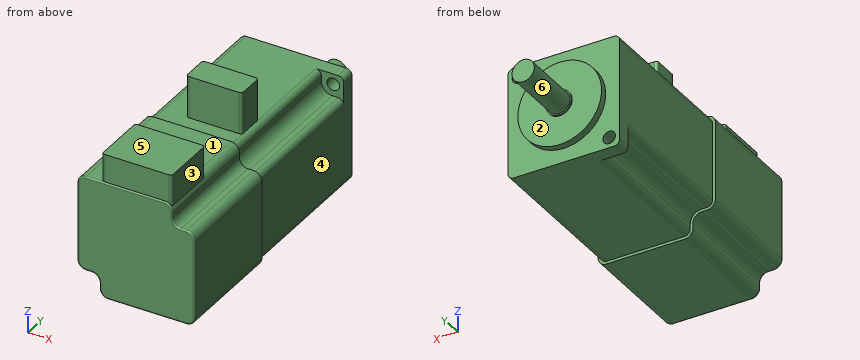
```python
from build123d import *

# Parameters (mm, degrees)
BOSS_EXTRUDE1_DEPTH             = 5
SKETCH2_R                       = 15
BOSS_EXTRUDE2_DEPTH             = 2.5
SKETCH3_R                       = 2.25
CUT_EXTRUDE1_DEPTH              = 5
BOSS_EXTRUDE3_DEPTH             = 51
BOSS_EXTRUDE4_DEPTH             = 40.5
SKETCH6_R                       = 4.5
BOSS_EXTRUDE5_DEPTH             = 0.5
SKETCH7_R                       = 4
BOSS_EXTRUDE6_DEPTH             = 21.5
FILLET1_R                       = 0.5
BOSS_EXTRUDE7_DEPTH             = 15
BOSS_EXTRUDE8_DEPTH             = 10
BOSS_EXTRUDE8_DIRECTION_2_REACH = 44


with BuildPart() as part:
    # Sketch1 → Boss-Extrude1 (new body)
    with BuildSketch(Plane(origin=(0, 0, 0), x_dir=(1, 0, 0), z_dir=(0, 1, 0))):
        with BuildLine():
            Line((2, 0), (38, 0))
            ThreePointArc((38, 0), (39.414213562, 0.585786438), (40, 2))
            Line((40, 2), (40, 38))
            ThreePointArc((40, 38), (39.414213562, 39.414213562), (38, 40))
            Line((38, 40), (2, 40))
            ThreePointArc((2, 40), (0.585786438, 39.414213562), (0, 38))
            Line((0, 38), (0, 2))
            ThreePointArc((0, 2), (0.585786438, 0.585786438), (2, 0))
        make_face()
    extrude(amount=BOSS_EXTRUDE1_DEPTH)

    # Sketch2 → Boss-Extrude2 (add)
    with BuildSketch(Plane(origin=(0, 5, 0), x_dir=(1, 0, 0), z_dir=(0, 1, 0))):
        with Locations((20, 20)):
            Circle(SKETCH2_R)
    extrude(amount=BOSS_EXTRUDE2_DEPTH)

    # Sketch3 → Cut-Extrude1 (cut)
    with BuildSketch(Plane(origin=(0, 5, 0), x_dir=(1, 0, 0), z_dir=(0, 1, 0))):
        with Locations((3.736544033, 36.263455967)):
            Circle(SKETCH3_R)
        with Locations((36.263455967, 3.736544033)):
            Circle(SKETCH3_R)
    extrude(amount=-CUT_EXTRUDE1_DEPTH, mode=Mode.SUBTRACT)

    # Sketch4 → Boss-Extrude3 (add)
    with BuildSketch(Plane.XZ):
        with BuildLine():
            Line((32, -2), (32, -4))
            ThreePointArc((32, -4), (33.171572875, -6.828427125), (36, -8))
            Line((36, -8), (38, -8))
            ThreePointArc((38, -8), (39.414213562, -8.585786438), (40, -10))
            Line((40, -10), (40, -38))
            ThreePointArc((40, -38), (39.414213562, -39.414213562), (38, -40))
            Line((38, -40), (10, -40))
            ThreePointArc((10, -40), (8.585786438, -39.414213562), (8, -38))
            Line((8, -38), (8, -36))
            ThreePointArc((8, -36), (6.828427125, -33.171572875), (4, -32))
            Line((4, -32), (2, -32))
            ThreePointArc((2, -32), (0.585786438, -31.414213562), (0, -30))
            Line((0, -30), (0, -2))
            ThreePointArc((0, -2), (0.585786438, -0.585786438), (2, 0))
            Line((2, 0), (30, 0))
            ThreePointArc((30, 0), (31.414213562, -0.585786438), (32, -2))
        make_face()
    extrude(amount=BOSS_EXTRUDE3_DEPTH)

    # Sketch5 → Boss-Extrude4 (add)
    with BuildSketch(Plane.XZ.offset(51)):
        with BuildLine():
            Line((10, -41), (38, -41))
            ThreePointArc((38, -41), (40.121320344, -40.121320344), (41, -38))
            Line((41, -38), (41, -10))
            ThreePointArc((41, -10), (40.121320344, -7.878679656), (38, -7))
            Line((38, -7), (36, -7))
            ThreePointArc((36, -7), (33.878679656, -6.121320344), (33, -4))
            Line((33, -4), (33, -2))
            ThreePointArc((33, -2), (32.121320344, 0.121320344), (30, 1))
            Line((30, 1), (2, 1))
            ThreePointArc((2, 1), (-0.121320344, 0.121320344), (-1, -2))
            Line((-1, -2), (-1, -30))
            ThreePointArc((-1, -30), (-0.121320344, -32.121320344), (2, -33))
            Line((2, -33), (4, -33))
            ThreePointArc((4, -33), (6.121320344, -33.878679656), (7, -36))
            Line((7, -36), (7, -38))
            ThreePointArc((7, -38), (7.878679656, -40.121320344), (10, -41))
        make_face()
    extrude(amount=BOSS_EXTRUDE4_DEPTH)

    # Sketch6 → Boss-Extrude5 (add)
    with BuildSketch(Plane(origin=(0, 7.5, 0), x_dir=(1, 0, 0), z_dir=(0, 1, 0))):
        with Locations((20, 20)):
            Circle(SKETCH6_R)
    extrude(amount=BOSS_EXTRUDE5_DEPTH)

    # Sketch7 → Boss-Extrude6 (add)
    with BuildSketch(Plane(origin=(0, 8, 0), x_dir=(1, 0, 0), z_dir=(0, 1, 0))):
        with Locations((20, 20)):
            Circle(SKETCH7_R)
    extrude(amount=BOSS_EXTRUDE6_DEPTH)

    # Fillet1
    fillet1_edges = [part.edges().sort_by_distance(p)[0] for p in [
        (7.878679656, -91.5, -40.121320344),
        (24, -91.5, -41),
        (40.121320344, -91.5, -40.121320344),
        (41, -91.5, -24),
        (40.121320344, -91.5, -7.878679656),
        (37, -91.5, -7),
        (33.878679656, -91.5, -6.121320344),
        (33, -91.5, -3),
        (32.121320344, -91.5, 0.121320344),
        (16, -91.5, 1),
        (-0.121320344, -91.5, 0.121320344),
        (-1, -91.5, -16),
        (-0.121320344, -91.5, -32.121320344),
        (3, -91.5, -33),
        (6.121320344, -91.5, -33.878679656),
        (7, -91.5, -37),
    ]]
    fillet(fillet1_edges, radius=FILLET1_R)

    # Sketch8 → Boss-Extrude7 (add)
    with BuildSketch(Plane.XY):
        with BuildLine():
            Line((11, -34.5), (29, -34.5))
            ThreePointArc((29, -34.5), (29.707106781, -34.792893219), (30, -35.5))
            Line((30, -35.5), (30, -43.5))
            ThreePointArc((30, -43.5), (29.707106781, -44.207106781), (29, -44.5))
            Line((29, -44.5), (11, -44.5))
            ThreePointArc((11, -44.5), (10.292893219, -44.207106781), (10, -43.5))
            Line((10, -43.5), (10, -35.5))
            ThreePointArc((10, -35.5), (10.292893219, -34.792893219), (11, -34.5))
        make_face()
    extrude(amount=BOSS_EXTRUDE7_DEPTH)

    # Sketch9 → Boss-Extrude8 (add)
    with BuildSketch(Plane.XY.offset(1)):
        with BuildLine():
            Line((8.5, -71), (31.5, -71))
            ThreePointArc((31.5, -71), (32.207106781, -71.292893219), (32.5, -72))
            Line((32.5, -72), (32.5, -90))
            ThreePointArc((32.5, -90), (32.207106781, -90.707106781), (31.5, -91))
            Line((31.5, -91), (8.5, -91))
            ThreePointArc((8.5, -91), (7.792893219, -90.707106781), (7.5, -90))
            Line((7.5, -90), (7.5, -72))
            ThreePointArc((7.5, -72), (7.792893219, -71.292893219), (8.5, -71))
        make_face()
    extrude(amount=BOSS_EXTRUDE8_DEPTH)

    # Sketch9 → Boss-Extrude8 direction 2 (add, up to next)
    with BuildSketch(Plane.XY.offset(1), mode=Mode.PRIVATE) as boss_extrude8_direction_2_sk1:
        with BuildLine():
            Line((8.5, -71), (31.5, -71))
            ThreePointArc((31.5, -71), (32.207106781, -71.292893219), (32.5, -72))
            Line((32.5, -72), (32.5, -90))
            ThreePointArc((32.5, -90), (32.207106781, -90.707106781), (31.5, -91))
            Line((31.5, -91), (8.5, -91))
            ThreePointArc((8.5, -91), (7.792893219, -90.707106781), (7.5, -90))
            Line((7.5, -90), (7.5, -72))
            ThreePointArc((7.5, -72), (7.792893219, -71.292893219), (8.5, -71))
        make_face()
    boss_extrude8_direction_2_tool1 = extrude(boss_extrude8_direction_2_sk1.sketch, amount=-BOSS_EXTRUDE8_DIRECTION_2_REACH, mode=Mode.PRIVATE) - part.part
    add(boss_extrude8_direction_2_tool1.solids().sort_by_distance((20, -81, 1))[0])


solid = part.part
```
Check sheet for the modelled part. Datum: model origin and axes. Units: mm. Face numbers are marked on the shaded views. A direction names the side the tool comes from. Give positions to 0.01 mm unless a question says otherwise; leave off trailing zeros. Loops run counter-clockwise (first coordinate to the right, second up) from the corner with the lowest first, then second, coordinate; pieces in that order, holes last. Notation, with made-up numbers: M 48,-33 L 90,-33 A24 cw 90,-9 Z; hole C 49.25,-28 d6. An arc over 180 degrees is marked long. Answer as CSV lines item,"result".
Item 1: Set-up check for the marked faces 4, 5 and 6: record each of +Z, -Z, +X, -X, +Y, -Y from which the full face is reachable in a straight line by a thin tool's end or side.
Reply:
face 4,"+Z, -Z, +X, +Y"
face 5,"+Z, +X, -X, -Y"
face 6,"+Y"
Item 2: Sectioned sample at A-A, the plane z = 6.5. Enter the section's corners in (x, y), then the cut area to 3 significant figures.
Reply:
outline,"M 7.5,-90 A1 ccw 8.5,-91 L 31.5,-91 A1 ccw 32.5,-90 L 32.5,-72 A1 ccw 31.5,-71 L 8.5,-71 A1 ccw 7.5,-72 Z; M 10,-43.5 A1 ccw 11,-44.5 L 29,-44.5 A1 ccw 30,-43.5 L 30,-35.5 A1 ccw 29,-34.5 L 11,-34.5 A1 ccw 10,-35.5 Z"
area,"698 mm^2"
Item 3: Depth check by flat-ended pin: pin 1 Ø12 at (x, y) = (6.5, -69) entering from +Z; pin 2 Ø7 at (x, z) = (36.26, -3.74) entering from +Y; pin 3 Ø1 at (x, y) = (36.5, -30) entering from +Z. Enter the tip coordinate at first touch or a pass-through.
Reply:
pin 1,"z = 11"
pin 2,"y = 5"
pin 3,"z = -8"
Item 4: Draft check along Y on the marked faces 1, 2 and 3. Enter one of: pulls with the +Y half, pulls with the -Y half, needs draft (parallel to the pull), parting line crosses it, or undercut.
Reply:
face 1,"undercut"
face 2,"pulls with the +Y half"
face 3,"needs draft"
Item 5: Scan lines: L1, parallel to Y at x = 18, z = 3.5; L2, parallel to Y at x = 4.5, z = -23; L3, parallel to Z at x = 38, y = -80. Record each from-to range of solid material in increasing order.
Reply:
L1,"-91 to -71, -44.5 to -34.5"
L2,"-91.5 to 5"
L3,"-41 to -7"
Item 6: Sectioned sample at B-B, the plane y = -75. Enter the section's corners in (x, z).
Reply:
outline,"M -1,-30 A3 ccw 2,-33 L 4,-33 A3 cw 7,-36 L 7,-38 A3 ccw 10,-41 L 38,-41 A3 ccw 41,-38 L 41,-10 A3 ccw 38,-7 L 36,-7 A3 cw 33,-4 L 33,-2 A3 ccw 32.5,-0.34 L 32.5,11 L 7.5,11 L 7.5,1 L 2,1 A3 ccw -1,-2 Z"
Item 7: Sectioned sample at D-D, the plane z = -20. Enter the section's corners in (x, y), then the cut area to 3 significant figures.
Reply:
outline,"M -1,-91 A0.5 ccw -0.5,-91.5 L 40.5,-91.5 A0.5 ccw 41,-91 L 41,-51 L 40,-51 L 40,5 L 35,5 L 35,7.5 L 24.5,7.5 L 24.5,8 L 24,8 L 24,29.5 L 16,29.5 L 16,8 L 15.5,8 L 15.5,7.5 L 5,7.5 L 5,5 L 0,5 L 0,-51 L -1,-51 Z"
area,"4,190 mm^2"
